```python
from build123d import *

# Parameters (mm, degrees)
SKETCH1_W          = 25
SKETCH1_H          = 25
SKETCH1_R          = 6
EXTRUDE1_DEPTH     = 5
SKETCH2_R          = 20.75
CUT_EXTRUDE1_DEPTH = 26


with BuildPart() as part:
    # Sketch1 → Extrude1 (new body)
    with BuildSketch(Plane(origin=(0, 0, 0), x_dir=(1, 0, 0), z_dir=(0, 1, 0))):
        with Locations((12.5, -12.5)):
            Rectangle(SKETCH1_W, SKETCH1_H)
        with Locations(Location((12, -12, 0), (0, 0, 270))):  # turned: the seam where the file's is
            Circle(SKETCH1_R, mode=Mode.SUBTRACT)
    extrude(amount=-EXTRUDE1_DEPTH)

    # Sketch2 → Cut-Extrude1 (cut, through all)
    with BuildSketch(Plane(origin=(0, 0, 0), x_dir=(0, 0, -1), z_dir=(1, 0, 0))):
        with Locations((-10, -21.5)):
            Circle(SKETCH2_R)
    extrude(amount=CUT_EXTRUDE1_DEPTH, mode=Mode.SUBTRACT)


solid = part.part
```
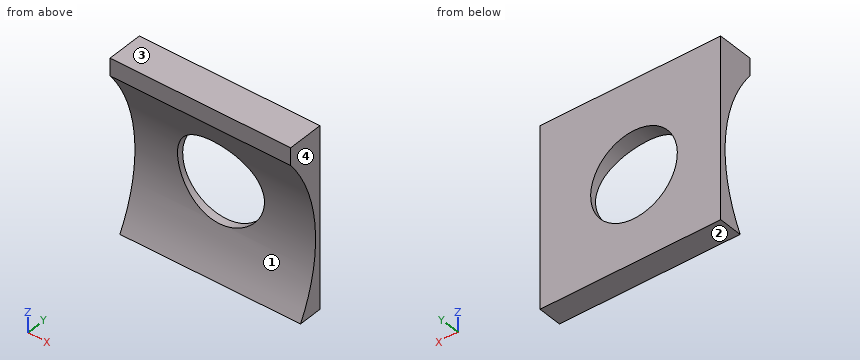
Here's how the part is built. I have some questions about the finished solid (model axes, mm). Face numbers are marked on the shaded views. Round coordinates to 2 decimals unless told otherwise and drop trailing zeros. Write each loop counter-clockwise with the first axis right and the second up, starting at its lowest first coordinate (ties: lowest second). Pieces come first, ordered by that corner, then holes.
Q1. If we section it at B-B on y = -2.05: Write out the boundary of the cut face in (x, z), plus the area to 3 significant figures.
Q2. If we section it at D-D on x = 4.5: Write out the boundary of the cut face in (y, z).
Q3. If we section it at A-A on x = 15: Write out the boundary of the cut face in (y, z), plus the area to 3 significant figures.
Q4. If we mould it in two halves opening along Z, with no side actions, what happens to the marked faces 1, 2, 3 and 4? For each: +Z half, -Z half, draft (parallel to the pull), parting line (faces both ways), or undercut.
Q5. If we section it at C-C on z = 13.5: Write out the boundary of the cut face in (x, y), plus the area to 3 significant figures.
Q6. Please list where these lines run through material, in increasing order: probe 1 along X at (y, z) = (-0.75, 12); probe 2 along Z at (x, y) = (14, -0.2).
Answer below:
1. outline: (0, 0) - (25, 0) - (25, 2.77) - (0, 2.77) - close; (0, 17.23) - (9.06, 17.23) arc R6 cw to (14.94, 17.23) - (25, 17.23) - (25, 25) - (0, 25) - close
1. area: 260 mm2
2. outline: (-5, 22.58) arc R20.75 cw to (-3.32, 0) - (0, 0) - (0, 25) - (-5, 25) - close
3. outline: (-5, 22.58) arc R20.75 cw to (-2.04, 17.2) - (0, 17.2) - (0, 25) - (-5, 25) - close; (-3.32, 0) - (0, 0) - (0, 6.8) - (-1, 6.8) arc R20.75 cw to start
3. area: 43.3 mm2
4. face 1: undercut
4. face 2: -Z half
4. face 3: +Z half
4. face 4: draft
5. outline: (0, -1.05) - (6.19, -1.05) - (6.19, 0) - (0, 0) - close; (17.81, -1.05) - (25, -1.05) - (25, 0) - (17.81, 0) - close
5. area: 14.0 mm2
6. probe 1: x = 0 to 6, 18 to 25
6. probe 2: z = 0 to 6.34, 17.66 to 25
